from build123d import *

# Parameters (mm, degrees)
BOSS_EXTRUDE1_DEPTH = 152.4
CUT_EXTRUDE1_DEPTH  = 69.58
CUT_EXTRUDE2_REACH  = 19.78
SKETCH4_W           = 30.48
SKETCH4_H           = 38.1


with BuildPart() as part:
    # Sketch2 → Boss-Extrude1 (new body)
    with BuildSketch(Plane.XY):
        with BuildLine():
            Line((0, 0), (68.58, 0))
            Line((68.58, 0), (49.587320143, 13.03542143))
            ThreePointArc((49.587320143, 13.03542143), (34.29, 17.78), (18.992679857, 13.03542143))
            Line((18.992679857, 13.03542143), (0, 0))
        make_face()
        with BuildLine():
            Line((10.997802271, 4.46752515), (8.189387654, 2.54))
            Line((8.189387654, 2.54), (9.965035751, 2.54))
            ThreePointArc((9.965035751, 2.54), (10.461920618, 3.514209799), (10.997802271, 4.46752515))
        make_face(mode=Mode.SUBTRACT)
        with BuildLine():
            Line((57.582197729, 4.46752515), (60.390612346, 2.54))
            Line((60.390612346, 2.54), (58.614964249, 2.54))
            ThreePointArc((58.614964249, 2.54), (58.118079382, 3.514209799), (57.582197729, 4.46752515))
        make_face(mode=Mode.SUBTRACT)
        with BuildLine():
            Line((12.82308193, 2.54), (55.75691807, 2.54))
            ThreePointArc((55.75691807, 2.54), (34.29, 15.24), (12.82308193, 2.54))
        make_face(mode=Mode.SUBTRACT)
    extrude(amount=BOSS_EXTRUDE1_DEPTH)

    # Sketch3 → Cut-Extrude1 (cut, through all)
    with BuildSketch(Plane(origin=(0, 0, 0), x_dir=(0, 0, -1), z_dir=(1, 0, 0))):
        Polygon((-17.78, 17.78), (0, 0), (0, 17.78), align=None)
    extrude(amount=CUT_EXTRUDE1_DEPTH, mode=Mode.SUBTRACT)

    # Sketch4 → Cut-Extrude2 (cut, up to next)
    with BuildSketch(Plane.XZ, mode=Mode.PRIVATE) as cut_extrude2_sk1:
        with Locations((34.29, 133.35)):
            Rectangle(SKETCH4_W, SKETCH4_H)
    cut_extrude2_tool1 = extrude(cut_extrude2_sk1.sketch, amount=-CUT_EXTRUDE2_REACH, mode=Mode.PRIVATE) & part.part
    add(cut_extrude2_tool1.solids().sort_by_distance((34.29, 0, 133.35))[0], mode=Mode.SUBTRACT)


solid = part.part
Design review of the part built by this model. Coordinates are the model's own, in mm. A direction names the side the tool comes from. Coordinates: 2 decimals unless noted, no trailing zeros. Order: outer loops, then holes, each group sorted by start corner. A loop starts at its lowest first (then second) coordinate and runs counter-clockwise, first axis right, second up. Notation, with made-up numbers: M -24,-4 L -15,-4 A25 cw -15,8 Z; hole C -35.5,33 d9. An arc over 180 degrees is marked long. Use a Markdown table: item, result.
(1) Wall thickness on probe 1 along X at (y, z) = (3.25, 16.5); probe 2 along Y at (x, z) = (34.5, 45); probe 3 along Y at (x, z) = (33, 109.5): over which ranges is each line inside the solid? List them lowest first.
Worked answers:
| item | result |
|---|---|
| probe 1 | x = 4.74 to 9.22, 10.32 to 13.23, 55.35 to 58.26, 59.36 to 63.84 |
| probe 2 | y = 0 to 2.54, 15.24 to 17.78 |
| probe 3 | y = 0 to 2.54, 15.21 to 17.75 |
(2) Add section A-A (x = 40.5). Give the boundary of the cut face in (y, z).
Worked answers:
| item | result |
|---|---|
| outline | M 0,0 L 2.54,2.54 L 2.54,114.3 L 0,114.3 Z; M 14.44,14.44 L 17.06,17.06 L 17.06,152.4 L 14.44,152.4 Z |
(3) Add section D-D (z = 122). Give the boundary of the cut face in (x, y).
Worked answers:
| item | result |
|---|---|
| outline | M 0,0 L 19.05,0 L 19.05,2.54 L 12.82,2.54 A24.49 cw 55.76,2.54 L 49.53,2.54 L 49.53,0 L 68.58,0 L 49.59,13.04 A27.03 ccw 18.99,13.04 Z; hole M 8.19,2.54 L 9.97,2.54 A27.03 cw 11,4.47 Z; hole M 57.58,4.47 A27.03 cw 58.61,2.54 L 60.39,2.54 Z |
(4) Draft analysis for pull direction Y (two halves, no side actions). For faces 1 (the flat face through (34, 0, 75)), 2 (the cylindrical face through (34.656, 15.237, 76.421)), 3 (the flat face through (34, 2, 2)), state which applies: released by +Y, released by -Y, zero draft, split by the parting line, or undercut.
Worked answers:
| item | result |
|---|---|
| face 1 | released by -Y |
| face 2 | undercut |
| face 3 | released by +Y |
(5) Add section B-B (y = 8). Give the boundary of the cut face in (x, z).
Worked answers:
| item | result |
|---|---|
| outline | M 11.66,8 L 16.9,8 L 16.9,152.4 L 11.66,152.4 Z; M 51.68,8 L 56.92,8 L 56.92,152.4 L 51.68,152.4 Z |
(6) For faces 4 (the flat face through (19.05, 1, 133)), 5 (the flat face through (59.217, 6.426, 75.133)), list the 3-axis set-ups (+Z, -Z, +X, -X, +Y, -Y) from which the entire face can be reached by the end or side of a thin tool; tool diameter is ignored.
Worked answers:
| item | result |
|---|---|
| face 4 | +Z, -Y |
| face 5 | +Z, -Z, +X, +Y |
(7) Add section C-C (z = 84). Give the boundary of the cut face in (x, y), then the cut area to 3 significant figures.
Worked answers:
| item | result |
|---|---|
| outline | M 0,0 L 68.58,0 L 49.59,13.04 A27.03 ccw 18.99,13.04 Z; hole M 8.19,2.54 L 9.97,2.54 A27.03 cw 11,4.47 Z; hole M 12.82,2.54 L 55.76,2.54 A24.49 ccw Z; hole M 57.58,4.47 A27.03 cw 58.61,2.54 L 60.39,2.54 Z |
| area | 354 mm2 |
(8) For P1, Ø10, axis at y = 9.5, z = 84, coming from the +X side; P2, Ø0.5, axis at x = 60, z = 82, coming from the +Y side; P3, Ø0.8, axis at x = 31, y = 1, coming from the +Z side; P4, Ø6, axis at x = 41.5, y = 11.5, coming from the +Z side, all flat-tipped, find the tip position at first contact; note any pin that passes through.
Worked answers:
| item | result |
|---|---|
| P1 | stops at x = 62.02 |
| P2 | stops at y = 6.06 |
| P3 | stops at z = 114.3 |
| P4 | stops at z = 152.4 |
